Read the model definition and answer for the solid it produces. Units are mm, in the model's axes. Round coordinates to 2 decimals unless told otherwise and drop trailing zeros. Write each loop counter-clockwise with the first axis right and the second up, starting at its lowest first coordinate (ties: lowest second). Pieces come first, ordered by that corner, then holes.
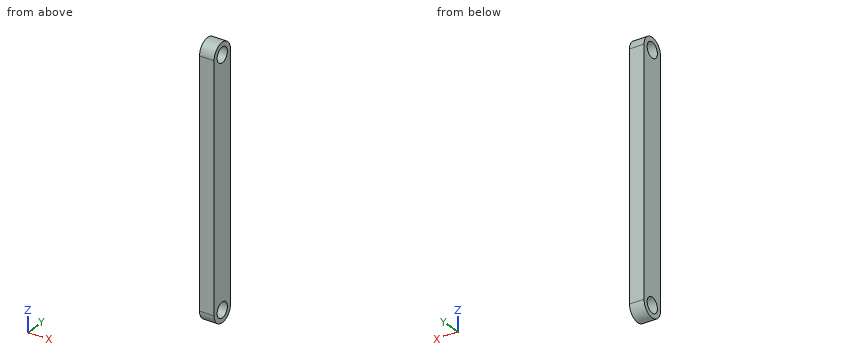
from build123d import *

# Parameters (mm, degrees)
F0_R     = 1.5625
F1_DEPTH = 3


with BuildPart() as f1:
    # F0 (on Right) → F1 (new body)
    with BuildSketch(Plane.YZ):
        with BuildLine():
            ThreePointArc((-5, 0), (-2.5, -2.5), (0, 0))
            Line((0, 0), (0, 50))
            ThreePointArc((0, 50), (-2.5, 52.5), (-5, 50))
            Line((-5, 50), (-5, 0))
        make_face()
        with Locations((-2.5, 0)):
            Circle(F0_R, mode=Mode.SUBTRACT)
        with Locations((-2.5, 50)):
            Circle(F0_R, mode=Mode.SUBTRACT)
    extrude(amount=F1_DEPTH)


solid = f1.part
Q1. Section A-A (y = -2.5) is taken. Determine the outline of the cut face in (x, z).
Verdict:
outline: (0, -2.5) - (3, -2.5) - (3, -1.56) - (0, -1.56) - close; (0, 1.56) - (3, 1.56) - (3, 48.44) - (0, 48.44) - close; (0, 51.56) - (3, 51.56) - (3, 52.5) - (0, 52.5) - close
Q2. Straight lines are drawn through the part: probe 1 along Z at (x, y) = (2.15, -2.5); probe 2 along Z at (x, y) = (0.3, -3.45); probe 3 along Z at (x, y) = (2.25, -0.75). For each, find the intervals that lie inside material, in ascending order.
Verdict:
probe 1: z = -2.5 to -1.56, 1.56 to 48.44, 51.56 to 52.5
probe 2: z = -2.31 to -1.24, 1.24 to 48.76, 51.24 to 52.31
probe 3: z = -1.79 to 51.79
Q3. Section B-B (x = 1.7) is taken. Determine the outline of the cut face in (y, z) (1 decimal), then the cut area to 3 significant figures.
Verdict:
outline: (-5, 0) arc R2.5 ccw to (0, 0) - (0, 50) arc R2.5 ccw to (-5, 50) - close; hole circle Ø3.1 at (-2.5, 0); hole circle Ø3.1 at (-2.5, 50)
area: 254 mm2
Q4. Flat-ended cylindrical pins translate along their axes: pin 1 Ø1.5 at (x, y) = (2.5, -3.5) entering from +Z; pin 2 Ø1 at (x, y) = (0.5, -1) entering from +Z. Find the tip coordinate at first contact, or state that the pin passes through.
Verdict:
pin 1: stops at z = 52.49
pin 2: stops at z = 52.29
